```python
from build123d import *
from build123d.topology import SkipClean

# Parameters (mm, degrees)
BOSS_EXTRUDE1_DEPTH = 500
BOSS_EXTRUDE2_START = 2
SKETCH3_R           = 73.2
SKETCH3_R_2         = 2
BOSS_EXTRUDE2_DEPTH = 2
SKETCH4_R           = 2
BOSS_EXTRUDE3_DEPTH = 2


with BuildPart() as part:
    # Sketch1 → Boss-Extrude1 (new body)
    with BuildSketch(Plane(origin=(0, 0, 0), x_dir=(1, 0, 0), z_dir=(0, 1, 0))):
        with BuildLine():
            ThreePointArc((-62.2, -38.592745432), (20.064894717, -70.396306721), (73.2, 0))
            ThreePointArc((73.2, 0), (-18.149380155, 70.914314493), (-64.2, -35.165323829))
            ThreePointArc((-64.2, -35.165323829), (-63.223229945, -36.892589978), (-62.2, -38.592745432))
        make_face()
        with BuildLine():
            ThreePointArc((-64.2, -30.786360616), (-66.88547387, -24.408469537), (-68.939103562, -17.8))
            Line((-68.939103562, -17.8), (-64.2, -17.8))
            Line((-64.2, -17.8), (-64.2, -30.786360616))
        make_face(mode=Mode.SUBTRACT)
        with BuildLine():
            Line((-62.2, -17.8), (62.2, -17.8))
            Line((62.2, -17.8), (62.2, -34.649675323))
            ThreePointArc((62.2, -34.649675323), (0, -71.2), (-62.2, -34.649675323))
            Line((-62.2, -34.649675323), (-62.2, -17.8))
        make_face(mode=Mode.SUBTRACT)
        with BuildLine():
            Line((64.2, -30.786360616), (64.2, -17.8))
            Line((64.2, -17.8), (68.939103562, -17.8))
            ThreePointArc((68.939103562, -17.8), (66.88547387, -24.408469537), (64.2, -30.786360616))
        make_face(mode=Mode.SUBTRACT)
        with BuildLine():
            Line((-64.2, -15.8), (-69.424779438, -15.8))
            ThreePointArc((-69.424779438, -15.8), (-70.756396664, 7.93551077), (-64.2, 30.786360616))
            Line((-64.2, 30.786360616), (-64.2, -15.8))
        make_face(mode=Mode.SUBTRACT)
        with BuildLine():
            ThreePointArc((-62.2, 34.649675323), (0, 71.2), (62.2, 34.649675323))
            Line((62.2, 34.649675323), (62.2, -15.8))
            Line((62.2, -15.8), (-62.2, -15.8))
            Line((-62.2, -15.8), (-62.2, 34.649675323))
        make_face(mode=Mode.SUBTRACT)
        with BuildLine():
            Line((64.2, -15.8), (64.2, 30.786360616))
            ThreePointArc((64.2, 30.786360616), (70.756396664, 7.93551077), (69.424779438, -15.8))
            Line((69.424779438, -15.8), (64.2, -15.8))
        make_face(mode=Mode.SUBTRACT)
    extrude(amount=BOSS_EXTRUDE1_DEPTH)

    # Sketch3 → Boss-Extrude2 (add)
    with SkipClean():  # the faces are left unmerged after this step: merging them gives an invalid solid
        with BuildSketch(Plane.XZ.offset(BOSS_EXTRUDE2_START)):
            with Locations(Location((0, 0, 0), (0, 0, 270))):
                Circle(SKETCH3_R)
            with Locations(Location((0, -27.7, 0), (0, 0, 270))):
                Circle(SKETCH3_R_2, mode=Mode.SUBTRACT)
            with Locations(Location((0, 41.5, 0), (0, 0, 270))):
                Circle(SKETCH3_R_2, mode=Mode.SUBTRACT)
        extrude(amount=-BOSS_EXTRUDE2_DEPTH)

    # Sketch4 → Boss-Extrude3 (add)
    # profile 1 of 2: a face of its own
    with SkipClean():  # the faces are left unmerged after this step: merging them gives an invalid solid
        with BuildSketch(Plane(origin=(0, 40, 0), x_dir=(1, 0, 0), z_dir=(0, 1, 0))):
            with BuildLine():
                Line((-62.2, -17.8), (-62.2, -34.649675323))
                ThreePointArc((-62.2, -34.649675323), (0, -71.2), (62.2, -34.649675323))
                Line((62.2, -34.649675323), (62.2, -17.8))
                Line((62.2, -17.8), (-62.2, -17.8))
            make_face()
            with Locations(Location((0, -41.5, 0), (0, 0, 90))):
                Circle(SKETCH4_R, mode=Mode.SUBTRACT)
        # profile 2 of 2: a face of its own
        with BuildSketch(Plane(origin=(0, 40, 0), x_dir=(1, 0, 0), z_dir=(0, 1, 0))):
            with BuildLine():
                Line((62.2, -15.8), (62.2, 34.649675323))
                ThreePointArc((62.2, 34.649675323), (0, 71.2), (-62.2, 34.649675323))
                Line((-62.2, 34.649675323), (-62.2, -15.8))
                Line((-62.2, -15.8), (62.2, -15.8))
            make_face()
            with Locations(Location((0, 27.7, 0), (0, 0, 90))):
                Circle(SKETCH4_R, mode=Mode.SUBTRACT)
        extrude(amount=BOSS_EXTRUDE3_DEPTH)


solid = part.part
```
The listing builds one solid part. Answer for the finished solid, in the listing's coordinates (mm). A direction names the side the tool comes from. Give positions to 0.01 mm unless a question says otherwise; leave off trailing zeros. Order: outer loops, then holes, each group sorted by start corner. A loop starts at its lowest first (then second) coordinate and runs counter-clockwise, first axis right, second up. Notation, with made-up numbers: (36, -39.5) -> (72, -39.5) arc R23 cw to (72, -29.5) -> close; hole circle Ø6 at (49.5, 30.25). An arc over 180 degrees is marked (long way). Answer as a JSON object with one key per item and string values. Group by question number.
Item 1: The part is cut by section D-D on x = -21.5. Write down the section's boundary in (y, z), and give its area (3 significant figures).
Item 2: The part is cut by section C-C on x = -50. Write down the section's boundary in (y, z), and give its area (3 significant figures).
Item 3: Flat-ended cylindrical pins translate along their axes: pin 1 (20 mm diameter, centred on y = 12.5, z = -11.5, fed in from -X); pin 2 (6.5 mm diameter, centred on x = 0, z = 41.5, fed in from +Y); pin 3 (8.5 mm diameter, centred on y = 14.5, z = 23, fed in from -X). Find the tip coordinate at first contact, or state that the pin passes through.
Item 4: Consider L1, parallel to Y at x = 29, z = -45; L2, parallel to Z at x = 24.5, y = 38.5; L3, parallel to Z at x = 31, y = 105.5. Determine where each line is inside the solid, lowest interval first. Write a range as from..to.
Item 5: A tool of negligible diameter and unlimited length cuts with its end or side. For faces 1 (the flat face through (-62.2, 268, -9)), 2 (the flat face through (62.2, 20, -10)), from which of +Z, -Z, +X, -X, +Y, -Y can it reach the whole face along a straight path? Write none if from no direction.
Item 6: The part is cut by section B-B on z = -53. Write down the section's boundary in (x, y).
Item 7: The part is cut by section A-A on y = 87. Write down the section's boundary in (x, z), and give its area (3 significant figures).
Result set:
{
 "1": {"outline": "(-2, -69.97) -> (500, -69.97) -> (500, -67.88) -> (42, -67.88) -> (42, 15.8) -> (500, 15.8) -> (500, 17.8) -> (42, 17.8) -> (42, 67.88) -> (500, 67.88) -> (500, 69.97) -> (-2, 69.97) -> close; hole (0, -67.88) -> (40, -67.88) -> (40, 15.8) -> (0, 15.8) -> close; hole (0, 17.8) -> (40, 17.8) -> (40, 67.88) -> (0, 67.88) -> close", "area": "3,640 mm²"},
 "2": {"outline": "(-2, -53.46) -> (500, -53.46) -> (500, -50.69) -> (42, -50.69) -> (42, 15.8) -> (500, 15.8) -> (500, 17.8) -> (42, 17.8) -> (42, 50.69) -> (500, 50.69) -> (500, 53.46) -> (-2, 53.46) -> close; hole (0, -50.69) -> (40, -50.69) -> (40, 15.8) -> (0, 15.8) -> close; hole (0, 17.8) -> (40, 17.8) -> (40, 50.69) -> (0, 50.69) -> close", "area": "4,190 mm²"},
 "3": {"pin 1": "x = -73.18", "pin 2": "y = 42", "pin 3": "x = -70.76"},
 "4": {"L1": "-2..0, 40..42", "L2": "-68.98..-66.85, 15.8..17.8, 66.85..68.98", "L3": "-66.31..-64.1, 15.8..17.8, 64.1..66.31"},
 "5": {"face 1": "+Y", "face 2": "none"},
 "6": {"outline": "(-50.49, -2) -> (50.49, -2) -> (50.49, 500) -> (47.54, 500) -> (47.54, 42) -> (-47.54, 42) -> (-47.54, 500) -> (-50.49, 500) -> close; hole (-47.54, 0) -> (47.54, 0) -> (47.54, 40) -> (-47.54, 40) -> close"},
 "7": {"outline": "circle Ø146.4 at (0, 0); hole (-69.42, 15.8) arc R71.2 ccw to (-64.2, -30.79) -> (-64.2, 15.8) -> close; hole (-68.94, 17.8) -> (-64.2, 17.8) -> (-64.2, 30.79) arc R71.2 ccw to start; hole (-62.2, -34.65) arc R71.2 ccw to (62.2, -34.65) -> (62.2, 15.8) -> (-62.2, 15.8) -> close; hole (-62.2, 17.8) -> (62.2, 17.8) -> (62.2, 34.65) arc R71.2 ccw to (-62.2, 34.65) -> close; hole (64.2, -30.79) arc R71.2 ccw to (69.42, 15.8) -> (64.2, 15.8) -> close; hole (64.2, 17.8) -> (68.94, 17.8) arc R71.2 ccw to (64.2, 30.79) -> close", "area": "1,440 mm²"}
}
